The listing builds one solid part. Answer for the finished solid, in the listing's coordinates (mm). Face numbers are marked on the shaded views. A direction names the side the tool comes from. Give positions to 0.01 mm unless a question says otherwise; leave off trailing zeros. Loops run counter-clockwise (first coordinate to the right, second up) from the corner with the lowest first, then second, coordinate; pieces in that order, holes last.
Item 1: Consider line 1 along Z through (x, y) = (12.7, 27); line 2 along Z through (x, y) = (270, 6); line 3 along Y through (x, z) = (97.75, 19.05) (3 decimals). Determine where each line is inside the solid, lowest interval first.
Item 2: Each of these flat-tipped pins is pushed along its axis until it touches: pin 1 Ø4 at (y, z) = (31, 85.5) entering from +X; pin 2 Ø4.5 at (y, z) = (44.45, 342.9) entering from -X; pin 3 Ø3 at (y, z) = (6.35, 342.9) entering from +X. Where does it stop, or does it pass through?
Item 3: Section D-D, the plane z = 136 is taken. Give the vertices of the cut face in (x, y), and give its area (3 significant figures).
Item 4: Section B-B, the plane z = 289.5 is taken. Give the vertices of the cut face in (x, y), and give its area (3 significant figures).
Item 5: Section A-A, the plane x = 12.7 is taken. Give the vertices of the cut face in (y, z), and give its area (3 significant figures).
Item 6: A tool of negligible diameter and unlimited length cuts with its end or side. For the marked faces 1 and 2, from which of +Z, -Z, +X, -X, +Y, -Y can it reach the whole face along a straight path? Write none if from no direction.
Item 7: Section C-C, the plane x = 243.5 is taken. Give the vertices of the cut face in (y, z).
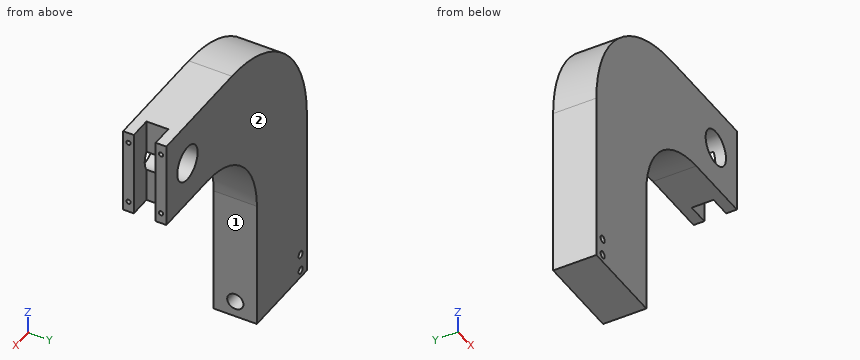
from build123d import *

# Parameters (mm, degrees)
F1_DEPTH  = 50.8
F3_D      = 8.334375
F5_D      = 19.05
F5_DEPTH  = 19.05
F5_TIP    = 5.7231973962
F6_W      = 25.654
F6_H      = 25.654
F7_DEPTH  = 355.601
F8_R      = 20.701
F9_DEPTH  = 50.801
F11_D     = 5.159375
F11_DEPTH = 25.4
F11_TIP   = 1.5500326281


with BuildPart() as f1:
    # F0 (on Front) → F1 (new body)
    with BuildSketch(Plane.XZ):
        with BuildLine():
            Line((0, 203.2), (0, 0))
            Line((0, 0), (101.6, 0))
            Line((101.6, 0), (101.6, 152.4))
            ThreePointArc((101.6, 152.4), (131.3579510314, 224.2420489686), (203.2, 254))
            Line((203.2, 254), (285.75, 254))
            Line((285.75, 254), (285.75, 355.6))
            Line((285.75, 355.6), (152.4, 355.6))
            ThreePointArc((152.4, 355.6), (44.6369265472, 310.9630734528), (0, 203.2))
        make_face()
    extrude(amount=-F1_DEPTH)

    # F3 (through all)
    with Locations(Plane.XZ):
        with Locations((12.7, 29.21), (12.7, 8.89)):
            Hole(F3_D / 2)

    # F5
    with Locations(Plane.YZ.offset(101.6)):
        with Locations((25.4, 19.05)):
            Hole(F5_D / 2, depth=F5_DEPTH)
            with Locations((0, 0, -(F5_DEPTH + F5_TIP / 2))):  # 118° drill point
                Cone(0, F5_D / 2, F5_TIP, mode=Mode.SUBTRACT)

    # F6 (on face) → F7 (cut, through all)
    with BuildSketch(Plane.XY.offset(355.6)):
        with Locations((272.923, 25.4)):
            Rectangle(F6_W, F6_H)
    extrude(amount=-F7_DEPTH, mode=Mode.SUBTRACT)

    # F8 (on face) → F9 (cut, through all)
    with BuildSketch(Plane.XZ):
        with Locations((242.9256, 304.8)):
            Circle(F8_R)
    extrude(amount=-F9_DEPTH, mode=Mode.SUBTRACT)

    # F11
    with Locations(Plane.YZ.offset(285.75)):
        with Locations((6.35, 342.9), (44.45, 342.9), (6.35, 266.7), (44.45, 266.7)):
            Hole(F11_D / 2, depth=F11_DEPTH)
            with Locations((0, 0, -(F11_DEPTH + F11_TIP / 2))):  # 118° drill point
                Cone(0, F11_D / 2, F11_TIP, mode=Mode.SUBTRACT)


solid = f1.part
Worked answers:
1. line 1: z = 0 to 4.72, 13.06 to 25.04, 33.38 to 264.11
1. line 2: z = 254 to 264.14, 269.26 to 340.34, 345.46 to 355.6
1. line 3: y = 0 to 15.875, 34.925 to 50.8
2. pin 1: stops at x = 101.6
2. pin 2: stops at x = 86.57
2. pin 3: stops at x = 259.7
3. outline: (0, 0) - (101.6, 0) - (101.6, 50.8) - (0, 50.8) - close
3. area: 5,160 mm2
4. outline: (26.79, 0) - (228.98, 0) - (228.98, 50.8) - (26.79, 50.8) - close; (256.87, 0) - (285.75, 0) - (285.75, 12.57) - (260.1, 12.57) - (260.1, 38.23) - (285.75, 38.23) - (285.75, 50.8) - (256.87, 50.8) - close
4. area: 11,100 mm2
5. outline: (0, 0) - (50.8, 0) - (50.8, 4.72) - (0, 4.72) - close; (0, 13.06) - (50.8, 13.06) - (50.8, 25.04) - (0, 25.04) - close; (0, 33.38) - (50.8, 33.38) - (50.8, 264.11) - (0, 264.11) - close
5. area: 12,600 mm2
6. face 1: -Z, +X, +Y, -Y
6. face 2: +Z, -Z, +X, -X, +Y
7. outline: (0, 254) - (50.8, 254) - (50.8, 284.11) - (0, 284.11) - close; (0, 325.49) - (50.8, 325.49) - (50.8, 355.6) - (0, 355.6) - close
